Can you work these out from the model? Positions are in its coordinate system, mm. A direction names the side the tool comes from. Coordinates: 2 decimals unless noted, no trailing zeros. Order: outer loops, then holes, each group sorted by start corner. A loop starts at its lowest first (then second) coordinate and runs counter-clockwise, first axis right, second up. Notation, with made-up numbers: (62.25, -1) -> (100.25, -1) arc R22 cw to (100.25, 8) -> close; hole circle Ø4 at (63, -30). An arc over 180 degrees is marked (long way). Answer in a Markdown table with one row per item. Add a question column.
1. Will these pins go through, and if not, where does the flat tip stop? pin 1 (8.5 mm diameter, centred on x = 12.7, y = -30, fed in from -Z); pin 2 (4 mm diameter, centred on x = 292.1, y = -30, fed in from +Z).
2. We'd pull the mould along Y, two halves only. Please class faces 3 (the face through (150, -30, 0)), 4 (the face through (138.5, -15.07, 3.04)), 5 (the face through (2.85, -56.99, 2.96)): pulls with the +Y half, pulls with the -Y half, needs draft (parallel to the pull), parting line crosses it, or undercut.
3. If I drill on line 1 along Y through (x, z) = (12.7, 4.7); line 2 along X through (y, z) = (-5, 2.7); line 3 along Y through (x, z) = (176, 2.1), over which ranges is the centre line in solid material (lowest first)? Write a range as [from, to].
4. Imagine slicing it at C-C on x = 96. Write out the boundary of the cut face in (y, z).
5. Imagine slicing it at D-D on z = 1.95. State how many separate pieces and enclosed holes the cut face has, plus the area to 3 significant figures.
6. Imagine slicing it at A-A on y = -36.5. Write out the boundary of the cut face in (x, z).
7. Imagine slicing it at B-B on x = 12.7. Write out the boundary of the cut face in (y, z).
8. On a 3-axis mill with a long thin cutter (end or side, diameter ignored), from which of +Z, -Z, +X, -X, +Y, -Y can I reach the whole of each face in a straight line? I mean faces 1 (the face through (304.8, -30, 3)), 2 (the face through (160.94, -44.93, 3.04)). Say none if no direction works.
from build123d import *

# Parameters (mm, degrees)
SKETCH001_R  = 3.25
PAD_DEPTH    = 6
POCKET_DEPTH = 6


with BuildPart() as part:
    # Sketch001 → Pad (new body)
    with BuildSketch(Plane.XY):
        with BuildLine():
            Line((0, -10), (0, -50))
            ThreePointArc((0, -50), (2.928932, -57.071068), (10, -60))
            Line((10, -60), (294.8, -60))
            ThreePointArc((294.8, -60), (301.871068, -57.071068), (304.8, -50))
            Line((304.8, -50), (304.8, -10))
            ThreePointArc((304.8, -10), (301.871068, -2.928932), (294.8, 0))
            Line((294.8, 0), (10, 0))
            ThreePointArc((10, 0), (2.928932, -2.928932), (0, -10))
        make_face()
        with Locations((292.1, -8)):
            Circle(SKETCH001_R, mode=Mode.SUBTRACT)
        with Locations((292.1, -52)):
            Circle(SKETCH001_R, mode=Mode.SUBTRACT)
        with Locations((292.1, -30)):
            Circle(SKETCH001_R, mode=Mode.SUBTRACT)
        with Locations((12.7, -8)):
            Circle(SKETCH001_R, mode=Mode.SUBTRACT)
        with Locations((12.7, -52)):
            Circle(SKETCH001_R, mode=Mode.SUBTRACT)
        with Locations((12.7, -30)):
            Circle(SKETCH001_R, mode=Mode.SUBTRACT)
    extrude(amount=PAD_DEPTH)

    # Sketch (on Face16 of Pad) → Pocket (cut)
    with BuildSketch(Plane.XY.offset(6)):
        Polygon((187.041016, -20), (169.720508, -10), (152.4, -20), (152.4, -40), (169.720508, -50), (187.041016, -40), align=None)
        Polygon((227.041016, -20), (209.720508, -10), (192.4, -20), (192.4, -40), (209.720508, -50), (227.041016, -40), align=None)
        Polygon((267.041016, -20), (249.720508, -10), (232.4, -20), (232.4, -40), (249.720508, -50), (267.041016, -40), align=None)
        Polygon((67.041016, -20), (49.720508, -10), (32.4, -20), (32.4, -40), (49.720508, -50), (67.041016, -40), align=None)
        Polygon((107.041016, -20), (89.720508, -10), (72.4, -20), (72.4, -40), (89.720508, -50), (107.041016, -40), align=None)
        Polygon((147.041016, -20), (129.720508, -10), (112.4, -20), (112.4, -40), (129.720508, -50), (147.041016, -40), align=None)
    extrude(amount=-POCKET_DEPTH, mode=Mode.SUBTRACT)


solid = part.part
Answers follow:
| question | item | result |
|---|---|---|
| 1 | pin 1 | stops at z = 0 |
| 1 | pin 2 | passes through |
| 2 | face 3 | needs draft |
| 2 | face 4 | undercut |
| 2 | face 5 | pulls with the -Y half |
| 3 | line 1 | y = [-60, -55.25], [-48.75, -33.25], [-26.75, -11.25], [-4.75, 0] |
| 3 | line 2 | x = [1.34, 11.45], [13.95, 290.85], [293.35, 303.46] |
| 3 | line 3 | y = [-60, -46.37], [-13.63, 0] |
| 4 | outline | (-60, 0) -> (-46.37, 0) -> (-46.37, 6) -> (-60, 6) -> close; (-13.63, 0) -> (0, 0) -> (0, 6) -> (-13.63, 6) -> close |
| 5 | separate pieces | 1 |
| 5 | enclosed holes | 12 |
| 5 | area | 11,800 mm² |
| 6 | outline | (0, 0) -> (32.4, 0) -> (32.4, 6) -> (0, 6) -> close; (67.04, 0) -> (72.4, 0) -> (72.4, 6) -> (67.04, 6) -> close; (107.04, 0) -> (112.4, 0) -> (112.4, 6) -> (107.04, 6) -> close; (147.04, 0) -> (152.4, 0) -> (152.4, 6) -> (147.04, 6) -> close; (187.04, 0) -> (192.4, 0) -> (192.4, 6) -> (187.04, 6) -> close; (227.04, 0) -> (232.4, 0) -> (232.4, 6) -> (227.04, 6) -> close; (267.04, 0) -> (304.8, 0) -> (304.8, 6) -> (267.04, 6) -> close |
| 7 | outline | (-60, 0) -> (-55.25, 0) -> (-55.25, 6) -> (-60, 6) -> close; (-48.75, 0) -> (-33.25, 0) -> (-33.25, 6) -> (-48.75, 6) -> close; (-26.75, 0) -> (-11.25, 0) -> (-11.25, 6) -> (-26.75, 6) -> close; (-4.75, 0) -> (0, 0) -> (0, 6) -> (-4.75, 6) -> close |
| 8 | face 1 | +Z, -Z, +X, +Y, -Y |
| 8 | face 2 | +Z, -Z |
